```python
from build123d import *

# Parameters (mm, degrees)
SKETCH3_R               = 7
BOSS_EXTRUDE1_DEPTH     = 19
SKETCH4_W               = 8.92
SKETCH4_H               = 10.7
CUT_EXTRUDE1_DEPTH      = 9
CUT_EXTRUDE1_DEPTH_BACK = 4.46
SKETCH5_R               = 1.25
CUT_EXTRUDE2_DEPTH      = 14.46
CUT_EXTRUDE2_DEPTH_BACK = 14.46
FILLET1_R               = 1


with BuildPart() as part:
    # Sketch1 → Revolve1 (revolve)
    with BuildSketch(Plane.XY):
        with BuildLine():
            Line((0, 0), (-5.6, 0))
            Line((-5.6, 0), (-5.6, 2.32))
            Line((-5.6, 2.32), (-5.095, 2.32))
            Line((-5.095, 2.32), (-5.095, 3.32))
            Line((-5.095, 3.32), (-5.6, 3.32))
            Line((-5.6, 3.32), (-5.6, 4.32))
            Line((-5.6, 4.32), (-5.095, 4.32))
            Line((-5.095, 4.32), (-5.095, 5.32))
            Line((-5.095, 5.32), (-5.6, 5.32))
            Line((-5.6, 5.32), (-5.6, 66.104936914))
            ThreePointArc((-5.6, 66.104936914), (-5.347653972, 80.311032213), (-4.590934282, 94.499203254))
            Line((-4.590934282, 94.499203254), (-3.714065718, 106.820796746))
            ThreePointArc((-3.714065718, 106.820796746), (-2.957346028, 121.008967787), (-2.705, 135.215063086))
            Line((-2.705, 135.215063086), (-2.705, 151))
            Line((-2.705, 151), (-2.17, 151))
            Line((-2.17, 151), (-2.17, 152))
            Line((-2.17, 152), (-2.705, 152))
            Line((-2.705, 152), (-2.705, 153))
            Line((-2.705, 153), (-2.17, 153))
            Line((-2.17, 153), (-2.17, 154))
            Line((-2.17, 154), (-2.705, 154))
            Line((-2.705, 154), (-2.705, 163.795))
            ThreePointArc((-2.705, 163.795), (-1.912723843, 165.707723843), (0, 166.5))
            Line((0, 166.5), (0, 0))
        make_face()
    revolve(axis=Axis((0, 0, 0), (0, 1, 0)))

    # Sketch3 → Boss-Extrude1 (add)
    with BuildSketch(Plane.XZ):
        Circle(SKETCH3_R)
    extrude(amount=BOSS_EXTRUDE1_DEPTH)

    # Sketch4 → Cut-Extrude1 (cut, two sides)
    with BuildSketch(Plane(origin=(0, 0, 0), x_dir=(0, 0, -1), z_dir=(1, 0, 0))) as cut_extrude1_sk:
        with Locations((0, -13.65)):
            Rectangle(SKETCH4_W, SKETCH4_H)
    extrude(amount=CUT_EXTRUDE1_DEPTH, mode=Mode.SUBTRACT)
    extrude(cut_extrude1_sk.sketch, amount=-CUT_EXTRUDE1_DEPTH_BACK, mode=Mode.SUBTRACT)

    # Sketch5 → Cut-Extrude2 (cut, two sides)
    with BuildSketch(Plane.XY) as cut_extrude2_sk:
        with Locations((0, -12.7)):
            Circle(SKETCH5_R)
        Polygon((5.395220107, -6), (5.395220107, -15.933988373), (0.784672068, -20.544536411), (9.016530708, -20.544536411), (9.016530708, -2.378689399), align=None)
    extrude(amount=CUT_EXTRUDE2_DEPTH, mode=Mode.SUBTRACT)
    extrude(cut_extrude2_sk.sketch, amount=-CUT_EXTRUDE2_DEPTH_BACK, mode=Mode.SUBTRACT)

    # Fillet1
    fillet1_edges = [part.edges().sort_by_distance(p)[0] for p in [
        (5.395220107, -6, 0),
        (2.329208479, -19, -5.530560099),
        (2.329208479, -19, 5.530560099),
        (-4.46, -13.65, -4.46),
        (-4.46, -13.65, 4.46),
    ]]
    fillet(fillet1_edges, radius=FILLET1_R)


solid = part.part
```
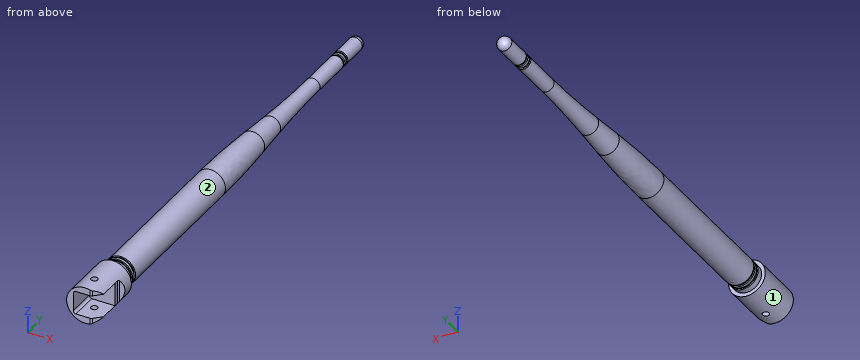
Verification items for the finished model (mm, model axes). Face numbers are marked on the shaded views. A direction names the side the tool comes from. Round coordinates to 2 decimals unless told otherwise and drop trailing zeros. Write each loop counter-clockwise with the first axis right and the second up, starting at its lowest first coordinate (ties: lowest second). Pieces come first, ordered by that corner, then holes. Notation, with made-up numbers: (32, 59.25) - (68, 59.25) arc R12 cw to (68, 73.25) - close; hole circle Ø5 at (-7.5, -6). An arc over 180 degrees is marked (long way). Answer as a JSON object with one key per item and string values. Group by question number.
Q1. Thickness scan on line 1 (X direction, y = -12.7, z = -6.1); line 2 (Y direction, x = 0, z = 6.5); line 3 (Z direction, x = 3.5, y = -9.5). Record the ranges inside material, lowest first.
Q2. Tool access check on the marked faces 1 and 2. Record the directions out of +Z, -Z, +X, -X, +Y, -Y that give a thin tool (end or side, any length) a straight path to the whole face; none if there is none.
Q3. Section check B-B, the plane y = 32. Enter the section's corners in (x, z).
Q4. Go/stop test with flat-tipped pins: pin 1 Ø4 at (y, z) = (36.5, 2.5) entering from +X; pin 2 Ø5.5 at (y, z) = (-12, -0.5) entering from +X; pin 3 Ø6 at (y, z) = (78, 0) entering from -X; pin 4 Ø2 at (x, y) = (0, -12.7) entering from -Z. Record where each tip stops, or that it passes through.
Q5. Section check A-A, the plane y = 140. Enter the section's corners in (x, z) (3 decimals).
Found:
{
 "1": {"line 1": "x = -3.43 to -1.25, 1.25 to 3.43", "line 2": "y = -19 to -13.95, -11.45 to 0", "line 3": "z = -6.06 to -4.46, 4.46 to 6.06"},
 "2": {"face 1": "+Y, -Y", "face 2": "+Y"},
 "3": {"outline": "circle Ø11.2 at (0, 0)"},
 "4": {"pin 1": "stops at x = 5.58", "pin 2": "stops at x = -4.46", "pin 3": "stops at x = -5.5", "pin 4": "passes through"},
 "5": {"outline": "circle Ø5.41 at (0, 0)"}
}
